from build123d import *

# Parameters (mm, degrees)
F2_R = 0.5
F3_R = 0.5


with BuildPart() as f1:
    # F0 (on Front) → F1 (revolve)
    with BuildSketch(Plane.XZ):
        Polygon((-4, -2.349634), (0, -2.349634), (0, 10.650366), (-2.25, 10.650366), (-2.5, 8.6337), (-2.5, 8.0287), (-2.25, 8.0287), (-2.5, 7.373284), (-2.5, 6.919534), (-2.25, 6.919534), (-2.5, 6.163284), (-2.5, -0.349634), (-4, -0.349634), align=None)
    revolve(axis=Axis((0, 0, 3.269001), (0, 0, 1)))

    # F2
    f2_edges = [f1.edges().sort_by_distance(p)[0] for p in [
        (4, 0, -2.349634),
    ]]
    fillet(f2_edges, radius=F2_R)

    # F3
    f3_edges = [f1.edges().sort_by_distance(p)[0] for p in [
        (2.25, 0, 10.650366),
        (4, 0, -0.349634),
    ]]
    fillet(f3_edges, radius=F3_R)


solid = f1.part
Could you check a few things on this model? Use its own coordinates, in mm. A direction names the side the tool comes from. Give positions to 0.01 mm unless a question says otherwise; leave off trailing zeros. Order: outer loops, then holes, each group sorted by start corner. A loop starts at its lowest first (then second) coordinate and runs counter-clockwise, first axis right, second up. Notation, with made-up numbers: (33.25, 86) -> (71.25, 86) arc R19 cw to (71.25, 90) -> close; hole circle Ø10 at (46, 32). An arc over 180 degrees is marked (long way). Return JSON: item names as keys, results as strings.
1. Imagine slicing it at A-A on x = 0. List the corners of the cut face in (y, z) for me.
Answer list:
{"outline": "(-4, -1.85) arc R0.5 ccw to (-3.5, -2.35) -> (3.5, -2.35) arc R0.5 ccw to (4, -1.85) -> (4, -0.85) arc R0.5 ccw to (3.5, -0.35) -> (2.5, -0.35) -> (2.5, 6.16) -> (2.25, 6.92) -> (2.5, 6.92) -> (2.5, 7.37) -> (2.25, 8.03) -> (2.5, 8.03) -> (2.5, 8.63) -> (2.3, 10.21) arc R0.5 ccw to (1.81, 10.65) -> (-1.81, 10.65) arc R0.5 ccw to (-2.3, 10.21) -> (-2.5, 8.63) -> (-2.5, 8.03) -> (-2.25, 8.03) -> (-2.5, 7.37) -> (-2.5, 6.92) -> (-2.25, 6.92) -> (-2.5, 6.16) -> (-2.5, -0.35) -> (-3.5, -0.35) arc R0.5 ccw to (-4, -0.85) -> close"}
2. On a 3-axis mill with a long thin cutter (end or side, diameter ignored), from which of +Z, -Z, +X, -X, +Y, -Y can I reach the whole of each face in a straight line? I mean faces 1 (the cylindrical face through (0.867, 3.905, -1.357)), 2 (the cylindrical face through (0.54, 2.44, 8.33)). Say none if no direction works.
Answer list:
{"face 1": "+Z, -Z", "face 2": "+Z"}
3. Imagine slicing it at C-C on z = 2. List the corners of the cut face in (x, y) for me.
Answer list:
{"outline": "circle Ø5 at (0, 0)"}
4. I need wall thicknesses on line 1 (Z direction, x = 0.75, y = -2.5); line 2 (X direction, y = -0.5, z = 7.5); line 3 (Z direction, x = 0.75, y = -2). Which ranges of each line are inside material? Lowest first, please. Write a range as from..to.
Answer list:
{"line 1": "z = -2.35..-0.35", "line 2": "x = -2.4..2.4", "line 3": "z = -2.35..10.53"}
5. Imagine slicing it at D-D on z = 6.5. List the corners of the cut face in (x, y) for me.
Answer list:
{"outline": "circle Ø4.78 at (0, 0)"}
6. For pin 1 Ø1.5 at (x, z) = (-1.5, 5) entering from -Y; pin 2 Ø1.5 at (y, z) = (0.5, 6.5) entering from +X; pin 3 Ø2 at (x, y) = (1.5, -2) entering from +Z, each with a flat end and sliding along its axis, tell me the tip position at first contact or that it passes through.
Answer list:
{"pin 1": "stops at y = -2.38", "pin 2": "stops at x = 2.5", "pin 3": "stops at z = 10.65"}
